The model under review builds one solid part; all positions refer to its coordinate system, in mm. Face numbers are marked on the shaded views. A direction names the side the tool comes from. Give positions to 0.01 mm unless a question says otherwise; leave off trailing zeros. Order: outer loops, then holes, each group sorted by start corner. A loop starts at its lowest first (then second) coordinate and runs counter-clockwise, first axis right, second up. Notation, with made-up numbers: (59.5, 51.5) -> (109.5, 51.5) arc R19 cw to (109.5, 60.5) -> close; hole circle Ø5 at (4.5, -30.5). An arc over 180 degrees is marked (long way). Answer as a JSON object with one key per item and string values. Group by question number.
from build123d import *

# Parameters (mm, degrees)
IZIM1_R                          = 50
Y_KSEKLIK_EKSTR_ZYON1_DEPTH      = 50
Y_KSEKLIK_EKSTR_ZYON2_REACH      = 218.16
Y_KSEKLIK_EKSTR_ZYON2_END_RADIUS = 65
IZIM2_R                          = 45
SALIENTE_EXTRUIR1_DEPTH          = 90
CROQUIS2_R                       = 22.752579474
SALIENTE_EXTRUIR2_DEPTH          = 7
SALIENTE_EXTRUIR4_DEPTH          = 7
CROQUIS4_R                       = 6.913256955
SALIENTE_EXTRUIR5_DEPTH          = 200
CROQUIS5_R                       = 2.363211774
CROQUIS5_R_2                     = 2.015238115
CROQUIS5_R_3                     = 2.465720792
CROQUIS5_R_4                     = 2.259668923
CROQUIS5_R_5                     = 2.225924281
CROQUIS5_R_6                     = 2.025363273
CROQUIS5_R_7                     = 2.390624595
CORTAR_EXTRUIR1_DEPTH            = 170


with BuildPart() as part:
    # Çizim1 → Yükseklik-Ekstrüzyon1 (new, symmetric)
    with BuildSketch(Plane.XY):
        with BuildLine():
            Line((-80, -40), (-80, 40))
            Line((-80, 40), (-22.281665693, 61.061668614))
            ThreePointArc((-22.281665693, 61.061668614), (65, 0), (-22.281665693, -61.061668614))
            Line((-22.281665693, -61.061668614), (-80, -40))
        make_face()
        Circle(IZIM1_R, mode=Mode.SUBTRACT)
    extrude(amount=Y_KSEKLIK_EKSTR_ZYON1_DEPTH, both=True)

    # Yükseklik-Ekstrüzyon2: up to this cylinder (the profile starts outside it)
    y_kseklik_ekstr_zyon2_end = Plane(origin=(0, 0, 0), z_dir=(0, 0, -1)) * Cylinder(Y_KSEKLIK_EKSTR_ZYON2_END_RADIUS, 567.32, mode=Mode.PRIVATE)
    # Çizim2 → Yükseklik-Ekstrüzyon2 (add, up to the surface)
    with BuildSketch(Plane(origin=(120, 0, 0), x_dir=(0, 0, -1), z_dir=(1, 0, 0)), mode=Mode.PRIVATE) as y_kseklik_ekstr_zyon2_sk1:
        Circle(IZIM2_R)
    y_kseklik_ekstr_zyon2_tool1 = extrude(y_kseklik_ekstr_zyon2_sk1.sketch, amount=-Y_KSEKLIK_EKSTR_ZYON2_REACH, mode=Mode.PRIVATE) - y_kseklik_ekstr_zyon2_end
    add(y_kseklik_ekstr_zyon2_tool1.solids().sort_by_distance((120, 0, 0))[0])

    # Croquis1 → Saliente-Extruir1 (add)
    with BuildSketch(Plane(origin=(120, 0, 0), x_dir=(0, 0, -1), z_dir=(1, 0, 0))):
        with BuildLine():
            Line((-43.760835361, 55.463261814), (43.760835361, 55.463261814))
            ThreePointArc((43.760835361, 55.463261814), (50.831903173, 52.534329626), (53.760835361, 45.463261814))
            Line((53.760835361, 45.463261814), (53.760835361, -45.463261814))
            ThreePointArc((53.760835361, -45.463261814), (50.831903173, -52.534329626), (43.760835361, -55.463261814))
            Line((43.760835361, -55.463261814), (-43.760835361, -55.463261814))
            ThreePointArc((-43.760835361, -55.463261814), (-50.831903173, -52.534329626), (-53.760835361, -45.463261814))
            Line((-53.760835361, -45.463261814), (-53.760835361, 45.463261814))
            ThreePointArc((-53.760835361, 45.463261814), (-50.831903173, 52.534329626), (-43.760835361, 55.463261814))
        make_face()
    extrude(amount=SALIENTE_EXTRUIR1_DEPTH)

    # Croquis2 → Saliente-Extruir2 (add)
    with BuildSketch(Plane(origin=(210, 0, 0), x_dir=(0, 0, -1), z_dir=(1, 0, 0))):
        Circle(CROQUIS2_R)
    extrude(amount=SALIENTE_EXTRUIR2_DEPTH)

    # Croquis3 → Saliente-Extruir4 (add)
    with BuildSketch(Plane(origin=(210, 0, 0), x_dir=(0, 0, -1), z_dir=(1, 0, 0))):
        Polygon((-34.126669907, 31.505010412), (-31.946398065, 36.408284276), (-35.102621872, 40.748092009), (-40.43911752, 40.18462588), (-42.619389362, 35.281352017), (-39.463165555, 30.941544283), align=None)
        Polygon((40.833645496, 31.505010412), (42.816653349, 36.749955525), (39.265901567, 41.089763259), (33.732141931, 40.18462588), (31.749134077, 34.939680767), (35.299885859, 30.599873033), align=None)
        Polygon((-33.036533986, -47.006056772), (-31.572165729, -41.257329502), (-35.818525457, -37.114785756), (-41.529253441, -38.720969281), (-42.993621697, -44.469696551), (-38.74726197, -48.612240297), align=None)
        Polygon((40.833645496, -47.809148535), (43.341315592, -42.261289535), (39.79056381, -37.315654026), (33.732141931, -37.917877518), (31.224471834, -43.465736518), (34.775223617, -48.411372026), align=None)
    extrude(amount=SALIENTE_EXTRUIR4_DEPTH)

    # Croquis4 → Saliente-Extruir5 (add)
    with BuildSketch(Plane(origin=(217, 0, 0), x_dir=(0, 0, -1), z_dir=(1, 0, 0))):
        Circle(CROQUIS4_R)
    extrude(amount=SALIENTE_EXTRUIR5_DEPTH)

    # Croquis5 → Cortar-Extruir1 (cut)
    with BuildSketch(Plane(origin=(417, 0, 0), x_dir=(0, 0, -1), z_dir=(1, 0, 0))):
        with Locations((-1.260150117, 6.797436533)):
            Circle(CROQUIS5_R)
        with Locations((2.849183045, -6.298831456)):
            Circle(CROQUIS5_R_2)
        with Locations((6.781038585, -1.345599286)):
            Circle(CROQUIS5_R_3)
        with Locations((4.68896459, 5.080032756)):
            Circle(CROQUIS5_R_4)
        with Locations((-3.582760742, -5.912440037)):
            Circle(CROQUIS5_R_5)
        with Locations((-6.781038585, -1.345599286)):
            Circle(CROQUIS5_R_6)
        with Locations((-5.942846302, 3.532095633)):
            Circle(CROQUIS5_R_7)
    extrude(amount=-CORTAR_EXTRUIR1_DEPTH, mode=Mode.SUBTRACT)


solid = part.part
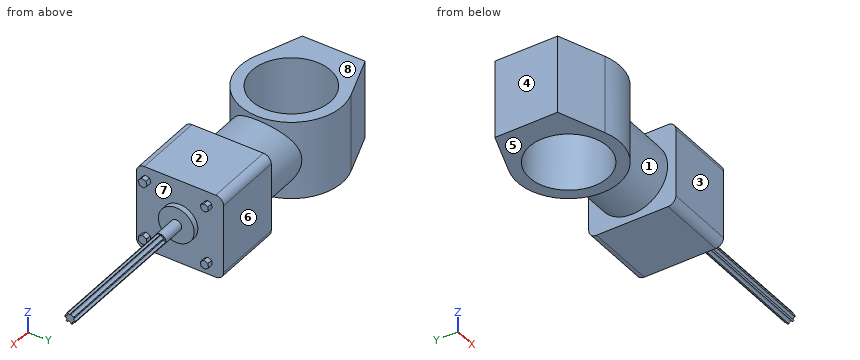
1. Take a section at B-B on x = 138. Give the boundary of the cut face in (y, z), plus the area to 3 significant figures.
2. For pin 1 (1.8 mm diameter, centred on y = 4.5, z = -4.5, fed in from +X); pin 2 (12.5 mm diameter, centred on y = -42, z = 36.5, fed in from +X); pin 3 (2 mm diameter, centred on x = 12, z = -9.5, fed in from +Y), all flat-tipped, find the tip position at first contact; note any pin that passes through.
3. Take a section at D-D on x = 72. Give the boundary of the cut face in (y, z), plus the area to 3 significant figures.
4. Machinability: for the marked faces 1, 2, 3, 4 and 5, which of the approach directions +Z, -Z, +X, -X, +Y, -Y give a long, thin tool a straight path to every point of the face, cutting with its end or side? Answer none if there is none.
5. Take a section at A-A on x = 0. Give the boundary of the cut face in (y, z).
6. For probe 1 along Y at (x, z) = (0, 9); probe 2 along X at (y, z) = (24, -16.5); probe 3 along X at (y, z) = (-7, -46), list the stretches that pass through material, from the lowest coordinate up. Write a range as [from, to].
7. Draft analysis for pull direction Y (two halves, no side actions). For the marked faces 6, 7 and 8, state which applies: pulls with the +Y half, pulls with the -Y half, needs draft (parallel to the pull), parting line crosses it, or undercut.
8. Take a section at C-C on z = 13. Give the boundary of the cut face in (x, y).
Checks:
{
 "1": {"outline": "(-55.46, -43.76) arc R10 ccw to (-45.46, -53.76) -> (45.46, -53.76) arc R10 ccw to (55.46, -43.76) -> (55.46, 43.76) arc R10 ccw to (45.46, 53.76) -> (-45.46, 53.76) arc R10 ccw to (-55.46, 43.76) -> close", "area": "11,800 mm2"},
 "2": {"pin 1": "stops at x = 247", "pin 2": "stops at x = 217", "pin 3": "stops at y = 64.06"},
 "3": {"outline": "circle Ø90 at (0, 0)", "area": "6,360 mm2"},
 "4": {"face 1": "none", "face 2": "+Z, +X, -X, +Y, -Y", "face 3": "+Z, -Z, +X, -Y", "face 4": "+Z, -Z, -X, +Y, -Y", "face 5": "-Z, -X, +Y, -Y"},
 "5": {"outline": "(-65, -50) -> (-50, -50) -> (-50, 50) -> (-65, 50) -> close; (50, -50) -> (65, -50) -> (65, 50) -> (50, 50) -> close"},
 "6": {"probe 1": "y = [-65, -50], [50, 65]", "probe 2": "x = [-80, -43.86], [43.86, 210]", "probe 3": "x = [-80, -49.51], [49.51, 64.62], [120, 210]"},
 "7": {"face 6": "pulls with the +Y half", "face 7": "undercut", "face 8": "needs draft"},
 "8": {"outline": "(-80, -40) -> (-22.28, -61.06) arc R65 ccw to (48.67, -43.08) -> (120, -43.08) -> (120, -55.46) -> (210, -55.46) -> (210, -18.67) -> (217, -18.67) -> (217, 18.67) -> (210, 18.67) -> (210, 55.46) -> (120, 55.46) -> (120, 43.08) -> (48.67, 43.08) arc R65 ccw to (-22.28, 61.06) -> (-80, 40) -> close; hole circle Ø100 at (0, 0)"}
}
